from build123d import *

# Parameters (mm, degrees)
SKETCH1_R           = 3.2639
BOSS_EXTRUDE1_DEPTH = 0.79375


with BuildPart() as part:
    # Sketch1 → Boss-Extrude1 (new, symmetric)
    with BuildSketch(Plane(origin=(0, 0, 0), x_dir=(0, 0, -1), z_dir=(1, 0, 0))):
        with BuildLine():
            Line((-44.152950291, -6.755130934), (-44.152950291, -8.484869066))
            Line((-44.152950291, -8.484869066), (-31.419145372, -7.896786517))
            Line((-31.419145372, -7.896786517), (-31.382526818, -8.689691394))
            Line((-31.382526818, -8.689691394), (-18.696048786, -8.103794532))
            Line((-18.696048786, -8.103794532), (-18.73266734, -7.310889655))
            Line((-18.73266734, -7.310889655), (0.297049709, -6.432044362))
            ThreePointArc((0.297049709, -6.432044362), (6.4389, 0), (0.297049709, 6.432044362))
            Line((0.297049709, 6.432044362), (-18.098343438, 7.281594812))
            Line((-18.098343438, 7.281594812), (-18.061724884, 8.074499689))
            Line((-18.061724884, 8.074499689), (-26.942259507, 8.484627492))
            Line((-26.942259507, 8.484627492), (-26.978878061, 7.691722615))
            Line((-26.978878061, 7.691722615), (-31.605185419, 7.905378364))
            ThreePointArc((-31.605185419, 7.905378364), (-34.50441496, -2.313203709), (-44.152950291, -6.755130934))
        make_face()
        Circle(SKETCH1_R, mode=Mode.SUBTRACT)
    extrude(amount=BOSS_EXTRUDE1_DEPTH, both=True)


solid = part.part
Here's how the part is built. I have some questions about the finished solid (model axes, mm). A direction names the side the tool comes from. Give positions to 0.01 mm unless a question says otherwise; leave off trailing zeros. Order: outer loops, then holes, each group sorted by start corner. A loop starts at its lowest first (then second) coordinate and runs counter-clockwise, first axis right, second up. Notation, with made-up numbers: M 62,16 L 119,16 A10 ccw 119,24 Z; hole C -0.5,86.25 d11. An arc over 180 degrees is marked long. Answer as a JSON object with one key per item and string values. Group by question number.
1) Suppose I cut it at D-D, the plane y = -4.75. Write out the boundary of the cut face in (x, z), plus the area to 3 significant figures.
2) Suppose I cut it at A-A, the plane y = 0. Write out the boundary of the cut face in (x, z).
3) On a 3-axis mill with a long thin cutter (end or side, diameter ignored), from which of +Z, -Z, +X, -X, +Y, -Y can I reach the whole of each face in a straight line? I mean faces 1 (the flat face through (0.011, -8.195, 37.875)), 2 (the flat face through (0.794, 0, 19)), 3 (the flat face through (0, 7.8, 29.3)). Say none if no direction works.
4) Suppose I cut it at B-B, the plane x = 0. Write out the boundary of the cut face in (y, z).
5) Suppose I cut it at C-C, the plane z = 38. Write out the boundary of the cut face in (x, y), plus the area to 3 significant figures.
6) We'd pull the mould along Z, two halves only. Please class faces 4 (the flat face through (-0.794, 0, 19)), 5 (the cylindrical face through (-0.011, -3.186, 0.708)), 6 (the flat face through (0, -8.4, 25.1)): pulls with the +Z half, pulls with the -Z half, needs draft (parallel to the pull), parting line crosses it, or undercut.
7) Please list where these lines run through material, in increasing order: L1, parallel to Z at x = -0.55, y = -3; L2, parallel to Z at x = -0.05, y = 1.5; L3, parallel to Y at x = -0.3, z = 2. Write a range as [from, to].
Results found:
{
 "1": {"outline": "M -0.79,-4.35 L 0.79,-4.35 L 0.79,37.3 L -0.79,37.3 Z", "area": "66.1 mm²"},
 "2": {"outline": "M -0.79,-6.44 L 0.79,-6.44 L 0.79,-3.26 L -0.79,-3.26 Z; M -0.79,3.26 L 0.79,3.26 L 0.79,32.93 L -0.79,32.93 Z"},
 "3": {"face 1": "+X, -X, -Y", "face 2": "+Z, -Z, +X, +Y, -Y", "face 3": "+X, -X, +Y"},
 "4": {"outline": "M -8.69,31.38 L -8.1,18.7 L -7.31,18.73 L -6.43,-0.3 A6.44 ccw 6.43,-0.3 L 7.28,18.1 L 8.07,18.06 L 8.48,26.94 L 7.69,26.98 L 7.91,31.61 A12.7 cw -6.76,44.15 L -8.48,44.15 L -7.9,31.42 Z; hole C 0,0 d6.53"},
 "5": {"outline": "M -0.79,-8.2 L 0.79,-8.2 L 0.79,-5.17 L -0.79,-5.17 Z", "area": "4.82 mm²"},
 "6": {"face 4": "needs draft", "face 5": "undercut", "face 6": "pulls with the -Z half"},
 "7": {"L1": "[-5.7, -1.29], [1.29, 35.14]", "L2": "[-6.26, -2.9], [2.9, 32.26]", "L3": "[-6.54, -2.58], [2.58, 6.54]"}
}
